Read the model definition and answer for the solid it produces. Units are mm, in the model's axes. A direction names the side the tool comes from. Coordinates: 2 decimals unless noted, no trailing zeros. Write each loop counter-clockwise with the first axis right and the second up, starting at its lowest first coordinate (ties: lowest second). Pieces come first, ordered by that corner, then holes. Notation, with made-up numbers: (48.25, 51) -> (52.25, 51) arc R18 cw to (52.25, 83) -> close; hole circle Ø2 at (3.25, 14.5). An arc over 180 degrees is marked (long way). One line per item, written item: value. Start each with the question number.
1. Find section B-B, the plane y = 37.5. Write down the section's boundary in (x, z).
2. Consider line 1 along Z through (x, y) = (-36, 35); line 2 along Y through (x, z) = (-28.5, -11). Determine where each line is inside the solid, lowest interval first.
3. Find section C-C, the plane x = -10. Write down the section's boundary in (y, z).
4. Given P1, Ø24, axis at x = -16, y = 20, coming from the +Z side; P2, Ø5, axis at x = -2.52, y = 43.5, coming from the -Z side; P3, Ø3.5, axis at x = -27.02, y = 18.5, coming from the -Z side; P4, Ø1.6, axis at y = 33.5, z = -33, coming from the -X side, each flat-ended and moving along its own axis, determine where each tip first touches the part or whether it passes through.
5. For faces 1 (the flat face through (-15, 2, -6)), 2 (the flat face through (-27.021, 31, -33)), 3 (the flat face through (-15, 1, 20.811)), determine the directions among +Z, -Z, +X, -X, +Y, -Y from which every point of the face is accessible in a straight line to the end or side of a thin tool.
6. Find section A-A, the plane x = -3.5. Write down the section's boundary in (y, z), and give its area (3 significant figures).
7. Find section D-D, the plane z = -18. Write down the section's boundary in (x, y), and give its area (3 significant figures).
8. For a pull along X with two mould halves and no side action, classify faces 4 (the flat face through (-38.771, 1.6, -14.7)), 5 (the cylindrical face through (-24.875, 19.178, -33.175)), 6 (the flat face through (-15, 0, -7)), 7 (the cylindrical face through (-14.55, 17.75, -33.18)) as pulls with the +X half, pulls with the -X half, needs draft (parallel to the pull), parting line crosses it, or undercut.
```python
from build123d import *

# Parameters (mm, degrees)
SKETCH1_W           = 48
SKETCH1_H           = 55
BOSS_EXTRUDE1_DEPTH = 2
SKETCH2_W           = 48
SKETCH2_H           = 2
BOSS_EXTRUDE2_DEPTH = 53
CUT_EXTRUDE1_DEPTH  = 53
CUT_EXTRUDE2_DEPTH  = 53
SKETCH5_R           = 2.25
CUT_EXTRUDE3_DEPTH  = 53


with BuildPart() as part:
    # Sketch1 → Boss-Extrude1 (new body)
    with BuildSketch(Plane(origin=(0, 0, 0), x_dir=(1, 0, 0), z_dir=(0, 1, 0))):
        with Locations((-14.771122877, 6.689300827)):
            Rectangle(SKETCH1_W, SKETCH1_H)
    extrude(amount=BOSS_EXTRUDE1_DEPTH)

    # Sketch2 → Boss-Extrude2 (add)
    with BuildSketch(Plane(origin=(0, 2, 0), x_dir=(1, 0, 0), z_dir=(0, 1, 0))):
        with Locations((-14.771122877, 33.189300827)):
            Rectangle(SKETCH2_W, SKETCH2_H)
    extrude(amount=BOSS_EXTRUDE2_DEPTH)

    # Sketch3 → Cut-Extrude1 (cut)
    with BuildSketch(Plane.XY.offset(-32.189300827)):
        with BuildLine():
            Line((-14.771122877, 55), (-38.771122877, 55))
            Line((-38.771122877, 55), (-38.771122877, 31))
            ThreePointArc((-38.771122877, 31), (-31.741685625, 47.970562748), (-14.771122877, 55))
        make_face()
        with BuildLine():
            Line((9.228877123, 55), (-14.771122877, 55))
            ThreePointArc((-14.771122877, 55), (2.199439872, 47.970562748), (9.228877123, 31))
            Line((9.228877123, 31), (9.228877123, 55))
        make_face()
    extrude(amount=-CUT_EXTRUDE1_DEPTH, mode=Mode.SUBTRACT)

    # Sketch4 → Cut-Extrude2 (cut)
    with BuildSketch(Plane.XY.offset(-32.189300827)):
        with BuildLine():
            Line((-27.021122877, 25.950247531), (-27.021122877, 36.049752469))
            ThreePointArc((-27.021122877, 36.049752469), (-14.771122877, 44.25), (-2.521122877, 36.049752469))
            Line((-2.521122877, 36.049752469), (-2.521122877, 25.950247531))
            ThreePointArc((-2.521122877, 25.950247531), (-14.771122877, 17.75), (-27.021122877, 25.950247531))
        make_face()
    extrude(amount=-CUT_EXTRUDE2_DEPTH, mode=Mode.SUBTRACT)

    # Sketch5 → Cut-Extrude3 (cut)
    with BuildSketch(Plane.XY.offset(-32.189300827)):
        with Locations((-27.021122877, 43.49749975)):
            Circle(SKETCH5_R)
        with Locations((-2.521122877, 43.49749975)):
            Circle(SKETCH5_R)
        with Locations((-27.021122877, 18.50250025)):
            Circle(SKETCH5_R)
        with Locations((-2.521122877, 18.50250025)):
            Circle(SKETCH5_R)
    extrude(amount=-CUT_EXTRUDE3_DEPTH, mode=Mode.SUBTRACT)


solid = part.part
```
Answer block:
1. outline: (-37.87, -34.19) -> (-26.32, -34.19) -> (-26.32, -32.19) -> (-37.87, -32.19) -> close; (-3.23, -34.19) -> (8.33, -34.19) -> (8.33, -32.19) -> (-3.23, -32.19) -> close
2. line 1: z = -34.19 to -32.19
2. line 2: y = 0 to 2
3. outline: (0, -34.19) -> (18.64, -34.19) -> (18.64, -32.19) -> (2, -32.19) -> (2, 20.81) -> (0, 20.81) -> close; (43.36, -34.19) -> (54.52, -34.19) -> (54.52, -32.19) -> (43.36, -32.19) -> close
4. P1: stops at z = -32.19
4. P2: stops at z = -34.19
4. P3: passes through
4. P4: stops at x = -38.71
5. face 1: +Z, +X, -X, +Y
5. face 2: +Z, -Z
5. face 3: +Z, +X, -X, +Y, -Y
6. outline: (0, -34.19) -> (16.48, -34.19) -> (16.48, -32.19) -> (2, -32.19) -> (2, 20.81) -> (0, 20.81) -> close; (20.53, -34.19) -> (24.03, -34.19) -> (24.03, -32.19) -> (20.53, -32.19) -> close; (37.97, -34.19) -> (41.47, -34.19) -> (41.47, -32.19) -> (37.97, -32.19) -> close; (45.52, -34.19) -> (52.19, -34.19) -> (52.19, -32.19) -> (45.52, -32.19) -> close
6. area: 166 mm2
7. outline: (-38.77, 0) -> (9.23, 0) -> (9.23, 2) -> (-38.77, 2) -> close
7. area: 96.0 mm2
8. face 4: pulls with the -X half
8. face 5: undercut
8. face 6: needs draft
8. face 7: undercut
